Source: CAD feature listing. Evaluate the final solid. Frame: model axes, mm. A direction names the side the tool comes from. Round coordinates to 2 decimals unless told otherwise and drop trailing zeros. Order: outer loops, then holes, each group sorted by start corner. A loop starts at its lowest first (then second) coordinate and runs counter-clockwise, first axis right, second up. Notation, with made-up numbers: (82, 5) -> (116, 5) arc R29 ccw to (116, 33) -> close; hole circle Ø5 at (51, 58). An arc over 180 degrees is marked (long way). Write item = value, one per line. Start each with the question number.
(1) Cut plane C-C on x = 15. Return the cut outline in (y, z), then the cut area to 3 significant figures.
(2) Ray query, line 1 (Y direction, x = 63, z = 7); line 2 (X direction, y = -30.5, z = 6.75); line 3 (Y direction, x = 81, z = 3.2). Return the intervals inside material, ascending.
(3) Contact query for flat-ended pins moving along their axis: pin 1 Ø2 at (x, y) = (32.8, -30) entering from +Z; pin 2 Ø4 at (y, z) = (-19, 3) entering from +X; pin 3 Ø1.5 at (x, z) = (20, 2) entering from -Y. Output: stop coordinate, or through.
(4) Cut plane B-B on y = 15. Return the cut outline in (x, z), then the cut area to 3 significant figures.
(5) Draft query along Y for faces 4 (the face through (28.57, -34.4, 2.46)), 5 (the face through (68, -17, 3)), 6 (the face through (82.908, 15.601, 2.535)). Return one class per face: released by +Y, released by -Y, zero draft, split by the parting line, or undercut.
(6) Reachability of faces 1 (the face through (28, -17, 3)), 2 (the face through (47, 30, 2)), 3 (the face through (60.34, -30.9, 7.46)) from +Z, -Z, +X, -X, +Y, -Y: full face, straight path, thin tool, end or side. Return the list, or none.
(7) Cut plane A-A on z = 6.75. Return the cut outline in (x, y).
(8) Cut plane D-D on y = -30. Return the cut outline in (x, z).
from build123d import *

# Parameters (mm, degrees)
SZKIC1_W                    = 96
SZKIC1_H                    = 30
DODANIE_WYCI_GNI_CIE1_DEPTH = 5
SZKIC2_W                    = 40
SZKIC2_H                    = 35
DODANIE_WYCI_GNI_CIE2_DEPTH = 5
SZKIC3_R                    = 2
WYTNIJ_WYCI_GNI_CIE1_DEPTH  = 5
SZKIC4_R                    = 3
DODANIE_WYCI_GNI_CIE3_DEPTH = 5
SZKIC5_R                    = 1.3
WYTNIJ_WYCI_GNI_CIE2_DEPTH  = 7
ZAOKR_GLENIE1_R             = 2


with BuildPart() as part:
    # Szkic1 → Dodanie-wyciągnięcie1 (new body)
    with BuildSketch(Plane.XY):
        with Locations((48, 15)):
            Rectangle(SZKIC1_W, SZKIC1_H)
    extrude(amount=DODANIE_WYCI_GNI_CIE1_DEPTH)

    # Szkic2 → Dodanie-wyciągnięcie2 (add)
    with BuildSketch(Plane.XY.offset(5)):
        with Locations((48, -17.5)):
            Rectangle(SZKIC2_W, SZKIC2_H)
    extrude(amount=-DODANIE_WYCI_GNI_CIE2_DEPTH)

    # Szkic3 → Wytnij-wyciągnięcie1 (cut)
    with BuildSketch(Plane.XY.offset(5)):
        with Locations((15, 15)):
            Circle(SZKIC3_R)
        with Locations((81, 15)):
            Circle(SZKIC3_R)
    extrude(amount=-WYTNIJ_WYCI_GNI_CIE1_DEPTH, mode=Mode.SUBTRACT)

    # Szkic4 → Dodanie-wyciągnięcie3 (add)
    with BuildSketch(Plane.XY.offset(5)):
        with Locations(Location((32.8, -30, 0), (0, 0, 180))):
            Circle(SZKIC4_R)
        with Locations(Location((63.2, -30, 0), (0, 0, 180))):
            Circle(SZKIC4_R)
        with Locations(Location((63.2, 21, 0), (0, 0, 180))):
            Circle(SZKIC4_R)
        with Locations(Location((32.8, 21, 0), (0, 0, 180))):
            Circle(SZKIC4_R)
    extrude(amount=DODANIE_WYCI_GNI_CIE3_DEPTH)

    # Szkic5 → Wytnij-wyciągnięcie2 (cut)
    with BuildSketch(Plane.XY.offset(10)):
        with Locations((32.8, 21)):
            Circle(SZKIC5_R)
        with Locations((63.2, 21)):
            Circle(SZKIC5_R)
        with Locations((32.8, -30)):
            Circle(SZKIC5_R)
        with Locations((63, -30)):
            Circle(SZKIC5_R)
    extrude(amount=-WYTNIJ_WYCI_GNI_CIE2_DEPTH, mode=Mode.SUBTRACT)

    # Zaokrąglenie1
    zaokr_glenie1_edges = [part.edges().sort_by_distance(p)[0] for p in [
        (28, -35, 2.5),
        (68, -35, 2.5),
    ]]
    fillet(zaokr_glenie1_edges, radius=ZAOKR_GLENIE1_R)


solid = part.part
Evaluation:
q1.outline = (0, 0) -> (13, 0) -> (13, 5) -> (0, 5) -> close; (17, 0) -> (30, 0) -> (30, 5) -> (17, 5) -> close
q1.area = 130 mm^2
q2.line_1 = -32.99 to -31.3, -28.7 to -27.01, 18.01 to 19.72, 22.28 to 23.99
q2.line_2 = 29.84 to 31.6, 34 to 35.76, 60.24 to 61.8, 64.2 to 66.16
q2.line_3 = 0 to 13, 17 to 30
q3.pin_1 = 3
q3.pin_2 = 68
q3.pin_3 = 0
q4.outline = (0, 0) -> (13, 0) -> (13, 5) -> (0, 5) -> close; (17, 0) -> (79, 0) -> (79, 5) -> (17, 5) -> close; (83, 0) -> (96, 0) -> (96, 5) -> (83, 5) -> close
q4.area = 440 mm^2
q5.face_4 = released by -Y
q5.face_5 = zero draft
q5.face_6 = undercut
q6.face_1 = +Z, -Z, -X, -Y
q6.face_2 = +Z, -Z, +X, -X, +Y
q6.face_3 = +Z
q7.outline = circle Ø6 at (32.8, -30); circle Ø6 at (32.8, 21); circle Ø6 at (63.2, -30); circle Ø6 at (63.2, 21); hole circle Ø2.6 at (32.8, -30); hole circle Ø2.6 at (32.8, 21); hole circle Ø2.6 at (63, -30); hole circle Ø2.6 at (63.2, 21)
q8.outline = (28, 0) -> (68, 0) -> (68, 5) -> (66.2, 5) -> (66.2, 10) -> (64.3, 10) -> (64.3, 3) -> (61.7, 3) -> (61.7, 10) -> (60.2, 10) -> (60.2, 5) -> (35.8, 5) -> (35.8, 10) -> (34.1, 10) -> (34.1, 3) -> (31.5, 3) -> (31.5, 10) -> (29.8, 10) -> (29.8, 5) -> (28, 5) -> close
